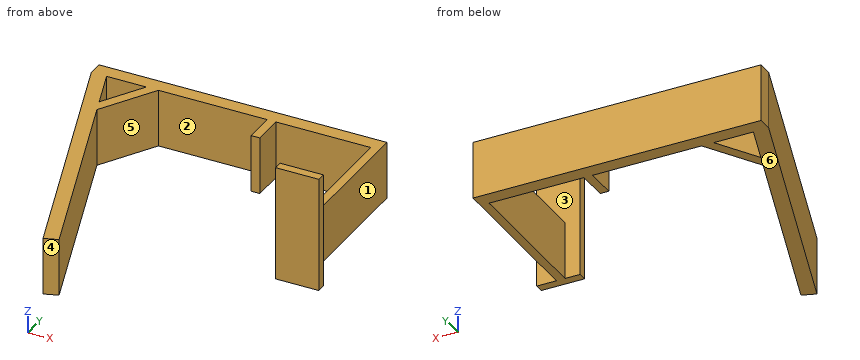
```python
from build123d import *

# Parameters (mm, degrees)
F0_W     = 3
F0_H     = 50.536646
F0_H_2   = 10.719895
F1_DEPTH = 20
F2_W     = 15
F2_H     = 40
F3_DEPTH = 3


with BuildPart() as f1:
    # F0 (on Top) → F1 (new body)
    with BuildSketch(Plane.XY):
        Polygon((-32.92932, 0), (0, 0), (3, 0), (3, 5), (-97, 5), (-97, 0), (-91.712957, 0), (-77.947989, 0), (-73.732667, 0), (-35.92932, 0), align=None)
        with Locations((1.5, -25.268323)):
            Rectangle(F0_W, F0_H)
        with Locations((-34.42932, -5.359947)):
            Rectangle(F0_W, F0_H_2)
        Polygon((-85.19516, -18.964979), (-73.732667, 0), (-77.947989, 0), (-86.723201, -14.518805), align=None)
        Polygon((-91.712957, 0), (-97, 0), (-64.49833, -94.570828), (-59.769789, -92.945744), (-85.19516, -18.964979), (-86.723201, -14.518805), align=None)
    extrude(amount=F1_DEPTH)

    # F2 (on face) → F3 (join)
    with BuildSketch(Plane.XZ.offset(50.536646)):
        with Locations((2.331055, 20)):
            Rectangle(F2_W, F2_H)
    extrude(amount=F3_DEPTH)


solid = f1.part
```
Can you work these out from the model? Positions are in its coordinate system, mm. Face numbers are marked on the shaded views. A direction names the side the tool comes from. Give positions to 0.01 mm unless a question says otherwise; leave off trailing zeros. Order: outer loops, then holes, each group sorted by start corner. A loop starts at its lowest first (then second) coordinate and runs counter-clockwise, first axis right, second up. Notation, with made-up numbers: M 10,-5 L 64,-5 A27 cw 64,21 Z; hole C 62,39 d8. An arc over 180 degrees is marked long. One line per item, written item: value.
1) I want a section at D-D, the plane y = -39. List the corners of the cut face in (x, z) for me, plus the area to 3 significant figures.
Answer sheet:
outline: M -83.6,0 L -78.31,0 L -78.31,20 L -83.6,20 Z; M 0,0 L 3,0 L 3,20 L 0,20 Z
area: 166 mm^2
2) We'd pull the mould along X, two halves only. Please class the marked faces 4, 5 and 6: released by +X, released by -X, zero draft, split by the parting line, or undercut.
Answer sheet:
face 4: released by +X
face 5: undercut
face 6: zero draft
3) Please list where these lines run through material, in increasing order: line 1 along Y through (x, z) = (-3.5, 6); line 2 along X through (y, z) = (-39, 3); line 3 along Y through (x, z) = (2, 36).
Answer sheet:
line 1: y = -53.54 to -50.54, 0 to 5
line 2: x = -83.6 to -78.31, 0 to 3
line 3: y = -53.54 to -50.54
4) I want a section at B-B, the plane x = -80. List the corners of the cut face in (y, z) for me.
Answer sheet:
outline: M -49.47,0 L -34.08,0 L -34.08,20 L -49.47,20 Z; M -10.37,0 L -3.4,0 L -3.4,20 L -10.37,20 Z; M 0,0 L 5,0 L 5,20 L 0,20 Z
5) I want a section at C-C, the plane y = -9. List the corners of the cut face in (x, z) for me, plus the area to 3 significant figures.
Answer sheet:
outline: M -93.91,0 L -88.62,0 L -88.62,20 L -93.91,20 Z; M -83.39,0 L -79.17,0 L -79.17,20 L -83.39,20 Z; M -35.93,0 L -32.93,0 L -32.93,20 L -35.93,20 Z; M 0,0 L 3,0 L 3,20 L 0,20 Z
area: 310 mm^2
6) I want a section at A-A, the plane z = 7.5. List the corners of the cut face in (x, y) for me.
Answer sheet:
outline: M -97,0 L -64.5,-94.57 L -59.77,-92.95 L -85.2,-18.96 L -73.73,0 L -35.93,0 L -35.93,-10.72 L -32.93,-10.72 L -32.93,0 L 0,0 L 0,-50.54 L -5.17,-50.54 L -5.17,-53.54 L 9.83,-53.54 L 9.83,-50.54 L 3,-50.54 L 3,5 L -97,5 Z; hole M -91.71,0 L -86.72,-14.52 L -77.95,0 Z
7) For P1, Ø5.5, axis at y = -6.5, z = 5, coming from the +X side; P2, Ø1, axis at y = -73.5, z = 20, coming from the +X side; P3, Ø12, axis at x = 3, z = 15.5, coming from the -Y side, each with a flat end and sliding along its axis, tell me the tip position at first contact or that it passes through.
Answer sheet:
P1: stops at x = 3
P2: stops at x = -66.28
P3: stops at y = -53.54
8) On a 3-axis mill with a long thin cutter (end or side, diameter ignored), from which of +Z, -Z, +X, -X, +Y, -Y can I reach the whole of each face in a straight line? I mean the marked faces 1, 2 and 3. Say none if no direction works.
Answer sheet:
face 1: +Z, -Z, +X, +Y
face 2: +Z, -Z
face 3: +Z
